Geometry: final body of the model. Coordinates: model frame, mm. A direction names the side the tool comes from. Give positions to 0.01 mm unless a question says otherwise; leave off trailing zeros. Write each loop counter-clockwise with the first axis right and the second up, starting at its lowest first coordinate (ties: lowest second). Pieces come first, ordered by that corner, then holes.
from build123d import *

# Parameters (mm, degrees)
F0_R     = 20
F1_DEPTH = 70
F2_R     = 2.5
F3_DEPTH = 320
F5_DEPTH = 3
F6_R     = 5


with BuildPart() as f1:
    # F0 (on Front) → F1 (new body)
    with BuildSketch(Plane.XZ):
        Circle(F0_R)
    extrude(amount=F1_DEPTH)

    # F2 (on face) → F3 (join)
    with BuildSketch(Plane(origin=(0, 0, 0), x_dir=(-1, 0, 0), z_dir=(0, 1, 0))):
        Circle(F2_R)
    extrude(amount=F3_DEPTH)

    # F4 (on face) → F5 (join)
    with BuildSketch(Plane(origin=(0, 320, 0), x_dir=(-1, 0, 0), z_dir=(0, 1, 0))):
        with BuildLine():
            Line((1.8400168651, 1.6924355043), (18.4001686511, 16.9243550427))
            ThreePointArc((18.4001686511, 16.9243550427), (10.0471668626, 22.8922353219), (0, 25))
            Line((0, 25), (0, 2.5))
            ThreePointArc((0, 2.5), (1.0047166863, 2.2892235322), (1.8400168651, 1.6924355043))
        make_face()
        with BuildLine():
            ThreePointArc((18.1144622727, -17.2298072122), (23.2148826921, -9.2773499229), (25, 0))
            Line((25, 0), (2.5, 0))
            ThreePointArc((2.5, 0), (2.3214882692, -0.9277349923), (1.8114462273, -1.7229807212))
            Line((1.8114462273, -1.7229807212), (18.1144622727, -17.2298072122))
        make_face()
        with BuildLine():
            ThreePointArc((-19.0723992016, -16.163031544), (-10.5100954182, -22.6834277458), (0, -25))
            Line((0, -25), (0, -2.5))
            ThreePointArc((0, -2.5), (-1.0510095418, -2.2683427746), (-1.9072399202, -1.6163031544))
            Line((-1.9072399202, -1.6163031544), (-19.0723992016, -16.163031544))
        make_face()
        with BuildLine():
            Line((-1.765668367, 1.7698630505), (-17.6566836704, 17.6986305053))
            ThreePointArc((-17.6566836704, 17.6986305053), (-23.0913088819, 9.5807856734), (-25, 0))
            Line((-25, 0), (-2.5, 0))
            ThreePointArc((-2.5, 0), (-2.3091308882, 0.9580785673), (-1.765668367, 1.7698630505))
        make_face()
    extrude(amount=-F5_DEPTH)

    # F6
    f6_edges = [f1.edges().sort_by_distance(p)[0] for p in [
        (-20, 0, 0),
    ]]
    fillet(f6_edges, radius=F6_R)


solid = f1.part
Q1. Pull-direction query (X, two-part tool) for faces 1 (the flat face through (16, 317, 7)), 2 (the flat face through (9.6, 318.52, 9.62)), 3 (the flat face through (-10, 318.5, 9.2)); classes: released by +X, released by -X, zero draft, split by the parting line, or undercut.
Filled sheet:
face 1: zero draft
face 2: undercut
face 3: released by -X
Q2. Access query for faces 4 (the flat face through (-9.85, 318.52, -9.37)), 5 (the cylindrical face through (-10.18, 318.521, 22.834)), 6 (the cylindrical face through (-4.336, -37.045, -19.524)), 7 (the flat face through (10.37, 318.52, -8.79)). Directions: +Z, -Z, +X, -X, +Y, -Y. A direction counts if a zero-diameter tool reaches every point of the face in a straight line with its end or side. Return the directions, or none.
Filled sheet:
face 4: -Z, +Y
face 5: +Z, -X, +Y, -Y
face 6: -Y
face 7: +X, +Y
Q3. Section A-A on y = 163.5. Output: boundary loops of the cut face in (x, z).
Filled sheet:
outline: circle Ø5 at (0, 0)
Q4. Section B-B on z = 9.5. Count the separate pieces of the cut face and the enclosed holes in it, plus the area to 3 significant figures.
Filled sheet:
separate pieces: 3
enclosed holes: 0
area: 2,520 mm2
Q5. Pin query (flat end, axial travel): P1, Ø3.5, axis at x = -11.5, y = 318, coming from the +Z side; P2, Ø5, axis at y = 48.5, z = 2.5, coming from the +X side; P3, Ø10, axis at y = -3.5, z = 7.5, coming from the -X side. Return the tip coordinate at first contact, or that it passes through.
Filled sheet:
P1: stops at z = 23.02
P2: stops at x = 2.5
P3: stops at x = -19.82
Q6. Ray query, line 1 along Y through (x, z) = (4, -14.5); line 2 along Y through (x, z) = (-21, -11); line 3 along Y through (x, z) = (-7.5, 6). Return the intervals inside material, ascending.
Filled sheet:
line 1: y = -70 to 0, 317 to 320
line 2: y = 317 to 320
line 3: y = -70 to 0
